from build123d import *

# Parameters (mm, degrees)
F1_DEPTH = 80
F2_R     = 2
F3_R     = 1


with BuildPart() as f1:
    # F0 (on Front) → F1 (new body)
    with BuildSketch(Plane.XZ):
        with BuildLine():
            Line((5, 25), (0, 25))
            Line((0, 25), (-2.952019, 8.258268))
            Line((-2.952019, 8.258268), (-12.800097, 9.99475))
            Line((-12.800097, 9.99475), (-13.106285, 8.258268))
            Line((-13.106285, 8.258268), (-13.106285, 5.7))
            Line((-13.106285, 5.7), (-14.462376, 5.7))
            ThreePointArc((-14.462376, 5.7), (-18.506285, 4.5), (-14.462376, 3.3))
            Line((-14.462376, 3.3), (-13.106285, 3.3))
            Line((-13.106285, 3.3), (-13.106285, 0))
            Line((-13.106285, 0), (-9.952019, 0))
            Line((-9.952019, 0), (-9.952019, 2.5))
            ThreePointArc((-9.952019, 2.5), (-7.452019, 5), (-4.952019, 2.5))
            Line((-4.952019, 2.5), (-4.952019, 0))
            Line((-4.952019, 0), (2.047981, 0))
            Line((2.047981, 0), (2.047981, 3.2))
            Line((2.047981, 3.2), (0.945348, 3.2))
            ThreePointArc((0.945348, 3.2), (-3.252019, 4.5), (0.945348, 5.8))
            Line((0.945348, 5.8), (2.047981, 5.8))
            Line((2.047981, 5.8), (2.047981, 8.258268))
            Line((2.047981, 8.258268), (5, 25))
        make_face()
    extrude(amount=F1_DEPTH)

    # F2
    f2_edges = [f1.edges().sort_by_distance(p)[0] for p in [
        (5, -40, 25),
        (-2.952019, -40, 8.258268),
    ]]
    fillet(f2_edges, radius=F2_R)

    # F3
    f3_edges = [f1.edges().sort_by_distance(p)[0] for p in [
        (0, -40, 25),
    ]]
    fillet(f3_edges, radius=F3_R)


solid = f1.part
The listing builds one solid part. Answer for the finished solid, in the listing's coordinates (mm). A direction names the side the tool comes from. Round coordinates to 2 decimals unless told otherwise and drop trailing zeros. Write each loop counter-clockwise with the first axis right and the second up, starting at its lowest first coordinate (ties: lowest second). Pieces come first, ordered by that corner, then holes. Notation, with made-up numbers: M 65,85 L 78,85 A26 ccw 78,111 Z; hole C 82.5,56.5 d8. An arc over 180 degrees is marked long. Write each question's results on one line, items separated by ' | '. Start each with the question number.
(1) The part is cut by section C-C, the plane z = 18.25. Write down the section's boundary in (x, y), and give its area (3 significant figures).
(2) Determine the mould class of faces 4 (the cylindrical face through (-7.5, -39.4, 5)), 5 (the flat face through (2.048, -39, 7)), 6 (the flat face through (-1.358, -39.44, 17.298)) for opening direction X: +X half, -X half, draft (parallel to the pull), parting line (faces both ways), or undercut.
(3) For faces 1 (the flat face through (-13.106, -39, 2)), 2 (the flat face through (-2, -39, 0)), 3 (the flat face through (-14, -39, 5.7)), determine the directions among +Z, -Z, +X, -X, +Y, -Y from which every point of the face is accessible in a straight line to the end or side of a thin tool.
(4) Each of these flat-tipped pins is pushed along its axis until it touches: P1, Ø1.6, axis at y = -42, z = 1, coming from the -X side; P2, Ø2.5, axis at y = -57.5, z = 2, coming from the +X side; P3, Ø1.5, axis at y = -56, z = 10, coming from the +X side. Where does it stop, or does it pass through?
(5) The part is cut by section B-B, the plane x = -8.75. Write down the section's boundary in (y, z).
(6) The part is cut by section A-A, the plane y = -41. Write down the section's boundary in (x, z).
(7) Find the intervals of material crossed by line 1 (Z direction, x = 1.25, y = -69); line 2 (Z direction, x = -2.75, y = -57.5); line 3 (X direction, y = -11, z = 8), in increasing order.
Worked answers:
1) outline: M -1.19,-80 L 3.81,-80 L 3.81,0 L -1.19,0 Z | area: 400 mm²
2) face 4: undercut | face 5: +X half | face 6: -X half
3) face 1: -Z, +Y, -Y | face 2: -Z, +X, -X, +Y, -Y | face 3: +Z, +Y, -Y
4) P1: stops at x = -13.11 | P2: stops at x = 2.05 | P3: stops at x = 2.49
5) outline: M -80,4.64 L 0,4.64 L 0,9.28 L -80,9.28 Z
6) outline: M -14.46,3.3 L -13.11,3.3 L -13.11,0 L -9.95,0 L -9.95,2.5 A2.5 cw -4.95,2.5 L -4.95,0 L 2.05,0 L 2.05,3.2 L 0.95,3.2 A2.3 cw long 0.95,5.8 L 2.05,5.8 L 2.05,8.26 L 4.59,22.65 A2 ccw 2.62,25 L 0.84,25 A1 ccw -0.15,24.17 L -2.6,10.23 A2 cw -4.92,8.61 L -12.8,9.99 L -13.11,8.26 L -13.11,5.7 L -14.46,5.7 A2.2 ccw long Z
7) line 1: z = 0 to 3.2, 5.8 to 25 | line 2: z = 0 to 3.07, 5.93 to 9.76 | line 3: x = -13.11 to 2.05
